Input: part model. Units: mm. Frame: model coordinates. A direction names the side the tool comes from. Round coordinates to 2 decimals unless told otherwise and drop trailing zeros. Order: outer loops, then holes, each group sorted by start corner. A loop starts at its lowest first (then second) coordinate and runs counter-clockwise, first axis right, second up. Notation, with made-up numbers: (89.25, 14.25) -> (139.25, 14.25) arc R8 cw to (139.25, 24.25) -> close; hole circle Ø5 at (-1.5, -25). An arc over 180 degrees is marked (long way). Use a Markdown table: item, result.
from build123d import *

# Parameters (mm, degrees)
SALIENTE_EXTRUIR1_DEPTH = 57
CROQUIS2_W              = 41
CROQUIS2_H              = 21
CORTAR_EXTRUIR1_DEPTH   = 40
CROQUIS3_R              = 1.5
CORTAR_EXTRUIR2_DEPTH   = 96.265502635
CROQUIS4_R              = 2.2
CORTAR_EXTRUIR3_DEPTH   = 95


with BuildPart() as part:
    # Croquis1 → Saliente-Extruir1 (new body)
    with BuildSketch(Plane(origin=(0, 0, 0), x_dir=(0, 0, -1), z_dir=(1, 0, 0))):
        Polygon((-1.684944658, 59.616081723), (-1.684944658, 70.445194562), (26.80274982, 58.606617394), (29.39371626, 46.700781546), align=None)
    extrude(amount=SALIENTE_EXTRUIR1_DEPTH)

    # Croquis2 → Cortar-Extruir1 (cut)
    with BuildSketch(Plane(origin=(0, 59.474011024, -24.71550197), x_dir=(1, 0, 0), z_dir=(0, 0.9234366793713986, -0.38375082956460804))):
        with Locations((28.5, -13.164518651)):
            Rectangle(CROQUIS2_W, CROQUIS2_H)
    extrude(amount=-CORTAR_EXTRUIR1_DEPTH, mode=Mode.SUBTRACT)

    # Croquis3 → Cortar-Extruir2 (cut, through all)
    with BuildSketch(Plane.ZY):
        with Locations((-20.337749265, 55.878708995)):
            Circle(CROQUIS3_R)
        with Locations((-4.419674199, 62.493753261)):
            Circle(CROQUIS3_R)
    extrude(amount=-CORTAR_EXTRUIR2_DEPTH, mode=Mode.SUBTRACT)

    # Croquis4 → Cortar-Extruir3 (cut)
    with BuildSketch(Plane(origin=(0, 59.474011024, -24.71550197), x_dir=(1, 0, 0), z_dir=(0, 0.9234366793713987, -0.3837508295646078))):
        with Locations(Location((4.6, -18.264518651, 0), (0, 0, 270))):
            Circle(CROQUIS4_R)
        with Locations(Location((4.6, -8.064518651, 0), (0, 0, 270))):
            Circle(CROQUIS4_R)
        with Locations(Location((52.4, -18.264518651, 0), (0, 0, 270))):
            Circle(CROQUIS4_R)
        with Locations(Location((52.4, -8.064518651, 0), (0, 0, 270))):
            Circle(CROQUIS4_R)
    extrude(amount=-CORTAR_EXTRUIR3_DEPTH, mode=Mode.SUBTRACT)


solid = part.part
1) Cut plane A-A on x = 31. Return loops of the section in (y, z), and give its area (3 significant figures).
Answer key:
| item | result |
|---|---|
| outline | (46.7, -29.39) -> (58.61, -26.8) -> (60.5, -22.25) -> (57.26, -20.91) arc R1.5 cw to (54.49, -19.76) -> (51.26, -18.42) -> close; (59.32, 0.97) -> (68.56, -2.86) -> (70.45, 1.68) -> (59.62, 1.68) -> close |
| area | 109 mm^2 |
2) Ray query, probe 1 along X at (y, z) = (59, -2); probe 2 along Z at (x, y) = (3, 59.5); probe 3 along X at (y, z) = (62.25, -6.5). Return the intervals inside material, ascending.
Answer key:
| item | result |
|---|---|
| probe 1 | x = 0 to 8, 49 to 57 |
| probe 2 | z = -24.65 to -17.63, -14.36 to -6.58, -3.31 to 1.41 |
| probe 3 | x = 0 to 2.43, 6.77 to 8, 49 to 50.23, 54.57 to 57 |
3) Cut plane B-B on z = -25.5. Return loops of the section in (x, y).
Answer key:
| item | result |
|---|---|
| outline | (0, 48.32) -> (57, 48.32) -> (57, 59.15) -> (0, 59.15) -> close |
4) Contact query for flat-ended pins moving along their axis: P1, Ø1.5, axis at x = 32.5, y = 59.5, coming from the -Z side; P2, Ø5, axis at x = 36.5, z = -21, coming from the -Y side; P3, Ø1, axis at x = 29.5, z = -5, coming from the +Y side. Output: stop coordinate, or through.
Answer key:
| item | result |
|---|---|
| P1 | stops at z = -26.46 |
| P2 | stops at y = 49.15 |
| P3 | passes through |
5) Set-up query: faces 4 (the face through (28.1, 54.97, -21.53)), 5 (the face through (28.2, 52.9, -19.1)). Return all of +Z, -Z, +X, -X, +Y, -Y with unobstructed straight access to the full face (end or side cutting, diameter ignored); none if empty.
Answer key:
| item | result |
|---|---|
| face 4 | +X, -X |
| face 5 | +Z, +Y |
6) Draft query along Z for faces 1 (the face through (26.26, 68.94, -1.94)), 2 (the face through (28.21, 58.9, -21.59)), 3 (the face through (0, 59, -14)). Return one class per face: released by +Z, released by -Z, zero draft, split by the parting line, or undercut.
Answer key:
| item | result |
|---|---|
| face 1 | released by -Z |
| face 2 | undercut |
| face 3 | zero draft |
7) Cut plane C-C on y = 48.75. Return loops of the section in (x, z), and give its area (3 significant figures).
Answer key:
| item | result |
|---|---|
| outline | (0, -28.95) -> (57, -28.95) -> (57, -24.46) -> (0, -24.46) -> close |
| area | 256 mm^2 |
